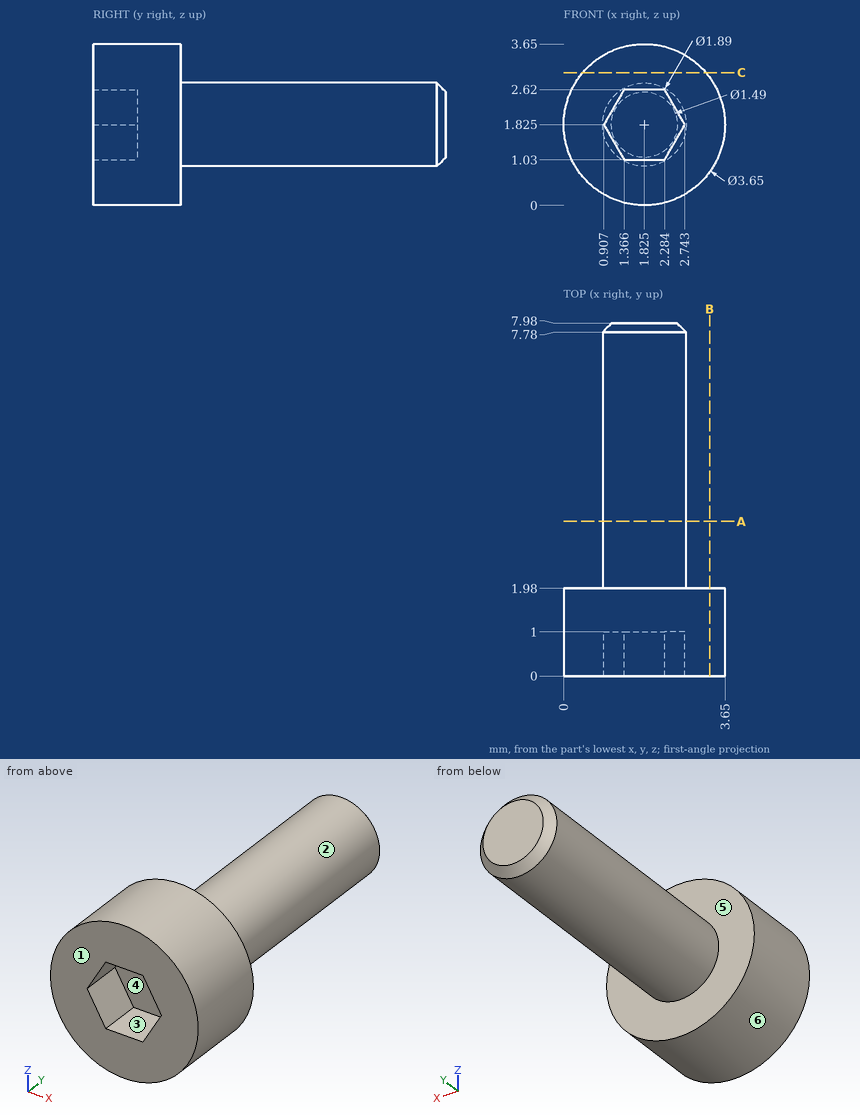
Drawing for the job (mm, zero at the part's lowest x, y, z). A direction names the side the tool comes from. Coordinates: 2 decimals unless noted, no trailing zeros. Order: outer loops, then holes, each group sorted by start corner. A loop starts at its lowest first (then second) coordinate and runs counter-clockwise, first axis right, second up. Notation, with made-up numbers: (81.25, 68.25) -> (106.25, 68.25) arc R27 cw to (106.25, 98.25) -> close; hole circle Ø7 at (6, -11.75). An arc over 180 degrees is marked (long way). Return JSON: item names as keys, results as strings.
Item 1: Slice it at A-A (y = 3.5). Write the cut outline in (x, z) (3 decimals), then the cut area to 3 significant figures.
Model answer:
{"outline": "circle Ø1.89 at (1.825, 1.825)", "area": "2.81 mm²"}
Item 2: Wall check: line 1 along Z through (x, y) = (1.9, 1.25); line 2 along Y through (x, z) = (1.4, 0.35); line 3 along X through (y, z) = (5.75, 2.05). Give the ranges that are in metal, low to high. Write a range as from..to.
Model answer:
{"line 1": "z = 0..3.65", "line 2": "y = 0..1.98", "line 3": "x = 0.91..2.74"}
Item 3: 3-axis set-ups, long thin cutter, end or side, ignore diameter. For the marked faces 1, 2 and 3: which of +Z, -Z, +X, -X, +Y, -Y reach the whole face in a straight line?
Model answer:
{"face 1": "+Z, -Z, +X, -X, -Y", "face 2": "+Y", "face 3": "-Y"}
Item 4: Mould opens along X. For the marked faces 4, 5 and 6 say: pulls with the +X half, pulls with the -X half, needs draft (parallel to the pull), parting line crosses it, or undercut.
Model answer:
{"face 4": "undercut", "face 5": "needs draft", "face 6": "parting line crosses it"}
Item 5: Slice it at C-C (z = 3). Write the cut outline in (x, y).
Model answer:
{"outline": "(0.43, 0) -> (3.22, 0) -> (3.22, 1.98) -> (0.43, 1.98) -> close"}
Item 6: Pin check, flat tips, straight feed: P1, Ø1.8, axis at x = 1, z = 1.5, coming from the +Y side; P2, Ø2, axis at x = 2.5, y = 4.5, coming from the -Z side; P3, Ø0.8, axis at x = 2, z = 2, coming from the -Y side. Stop position of each tip, or through.
Model answer:
{"P1": "stops at y = 7.98", "P2": "stops at z = 0.88", "P3": "stops at y = 1"}
Item 7: Slice it at B-B (x = 3.3). Write the cut outline in (y, z), then the cut area to 3 significant figures.
Model answer:
{"outline": "(0, 0.75) -> (1.98, 0.75) -> (1.98, 2.9) -> (0, 2.9) -> close", "area": "4.26 mm²"}
